from build123d import *


with BuildPart() as part:
    # Sketch1 → Revolve-Thin1 (revolve)
    with BuildSketch(Plane(origin=(0, 0, 0), x_dir=(0, 0, -1), z_dir=(1, 0, 0)), mode=Mode.PRIVATE) as revolve_thin1_sk:
        Polygon((0, 0), (-82.77987, 0), (-79.050134, 13.891514), (-50.756312, 13.891514), (-42.491914, 19.664934), (-40.819324, 80.659732), (0, 80.659732), (0, 78.119732), (-38.348020684, 78.119732), (-39.987956021, 18.315760551), (-49.9569701, 11.351514), (-77.102141701, 11.351514), (-79.467947256, 2.54), (0, 2.54), align=None)
    revolve(revolve_thin1_sk.sketch.rotate(Axis((0, 0, 0), (0, 1, 0)), 180), axis=Axis((0, 0, 0), (0, 1, 0)))


solid = part.part
Geometry: final body of the model. Coordinates: model frame, mm. A direction names the side the tool comes from. Give positions to 0.01 mm unless a question says otherwise; leave off trailing zeros. Write each loop counter-clockwise with the first axis right and the second up, starting at its lowest first coordinate (ties: lowest second). Pieces come first, ordered by that corner, then holes. Notation, with made-up numbers: (27.25, 20.25) - (32.25, 20.25) arc R16 cw to (32.25, 29.25) - close; hole circle Ø8 at (-26, 71). An arc over 180 degrees is marked (long way). Return JSON: item names as keys, results as strings. Group by question number.
1) Mould query, pull axis X, two halves, no side actions, for faces 4 (the flat face through (-1, 80.66, 1)), 5 (the conical face through (38.054, 19.385, -19.793)), 6 (the flat face through (-1, 2.54, 1)). Classes: released by +X, released by -X, zero draft, split by the parting line, or undercut.
2) First-contact query: P1, Ø12, axis at x = -24.5, y = 53.5, coming from the +Z side; P2, Ø1, axis at x = 42, z = 37.5, coming from the +Y side; P3, Ø2, axis at y = 35.5, z = -29.5, coming from the -X side. Flat tips, straight axial feed; report the tip coordinate or a pass-through.
3) Line query: line 1 (Y direction, x = 10, z = -12); line 2 (Y direction, x = 68.5, z = 1); line 3 (Z direction, x = 28, y = 58.5). Output: solid intervals per line, ascending.
4) Section B-B on x = 0. Return the cut outline in (y, z).
5) Section A-A on z = 0. Return the cut outline in (x, y), plus the area to 3 significant figures.
6) Set-up query: faces 1 (the flat face through (-1, 0, -1)), 2 (the conical face through (-38.846, 47.799, 5.1)), 3 (the conical face through (-12.51, 50.59, -39.72)). Return all of +Z, -Z, +X, -X, +Y, -Y with unobstructed straight access to the full face (end or side cutting, diameter ignored); none if empty.
7) Section C-C on y = 29. Return the cut outline in (x, z).
Filled in:
{
 "1": {"face 4": "zero draft", "face 5": "split by the parting line", "face 6": "undercut"},
 "2": {"P1": "stops at z = 37.23", "P2": "stops at y = 13.89", "P3": "stops at x = -30.93"},
 "3": {"line 1": "y = 0 to 2.54, 78.12 to 80.66", "line 2": "y = 0 to 2.54, 11.35 to 13.89", "line 3": "z = -30.53 to -26.98, 26.98 to 30.53"},
 "4": {"outline": "(0, -82.78) - (13.89, -79.05) - (13.89, -50.76) - (19.66, -42.49) - (80.66, -40.82) - (80.66, 40.82) - (19.66, 42.49) - (13.89, 50.76) - (13.89, 79.05) - (0, 82.78) - close; hole (2.54, -79.47) - (11.35, -77.1) - (11.35, -49.96) - (18.32, -39.99) - (78.12, -38.35) - (78.12, 38.35) - (18.32, 39.99) - (11.35, 49.96) - (11.35, 77.1) - (2.54, 79.47) - close"},
 "5": {"outline": "(-82.78, 0) - (82.78, 0) - (79.05, 13.89) - (50.76, 13.89) - (42.49, 19.66) - (40.82, 80.66) - (-40.82, 80.66) - (-42.49, 19.66) - (-50.76, 13.89) - (-79.05, 13.89) - close; hole (-79.47, 2.54) - (79.47, 2.54) - (77.1, 11.35) - (49.96, 11.35) - (39.99, 18.32) - (38.35, 78.12) - (-38.35, 78.12) - (-39.99, 18.32) - (-49.96, 11.35) - (-77.1, 11.35) - close", "area": "1,180 mm^2"},
 "6": {"face 1": "+Z, -Z, +X, -X, -Y", "face 2": "none", "face 3": "+Y"},
 "7": {"outline": "circle Ø84.47 at (0, 0); hole circle Ø79.39 at (0, 0)"}
}
